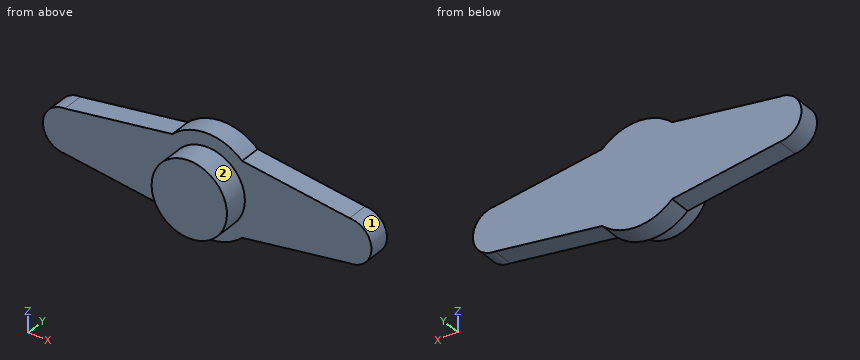
```python
from build123d import *

# Parameters (mm, degrees)
BOSS_EXTRUDE1_DEPTH = 2.54
SKETCH2_R           = 4.3688
BOSS_EXTRUDE2_DEPTH = 2.921


with BuildPart() as part:
    # Sketch1 → Boss-Extrude1 (new body)
    with BuildSketch(Plane(origin=(0, 0, 0), x_dir=(1, 0, 0), z_dir=(0, 1, 0))):
        with BuildLine():
            Line((4.047217222, 4.318), (16.51, 2.54))
            ThreePointArc((16.51, 2.54), (19.05, 0), (16.51, -2.54))
            Line((16.51, -2.54), (4.047217222, -4.318))
            ThreePointArc((4.047217222, -4.318), (0, -5.9182), (-4.047217222, -4.318))
            Line((-4.047217222, -4.318), (-16.51, -2.54))
            ThreePointArc((-16.51, -2.54), (-19.05, 0), (-16.51, 2.54))
            Line((-16.51, 2.54), (-4.047217222, 4.318))
            ThreePointArc((-4.047217222, 4.318), (0, 5.9182), (4.047217222, 4.318))
        make_face()
    extrude(amount=BOSS_EXTRUDE1_DEPTH)

    # Sketch2 → Boss-Extrude2 (add)
    with BuildSketch(Plane.XZ):
        with Locations(Location((0, 0, 0), (0, 0, 270))):
            Circle(SKETCH2_R)
    extrude(amount=BOSS_EXTRUDE2_DEPTH)


solid = part.part
```
For this review, take the finished solid that the model builds, in its own axes (mm). Face numbers are marked on the shaded views. A direction names the side the tool comes from. Round coordinates to 2 decimals unless told otherwise and drop trailing zeros. Write each loop counter-clockwise with the first axis right and the second up, starting at its lowest first coordinate (ties: lowest second). Pieces come first, ordered by that corner, then holes. Notation, with made-up numbers: (37.25, -7.75) - (87.25, -7.75) arc R23 cw to (87.25, 26.25) - close; hole circle Ø2 at (70.5, -27). An arc over 180 degrees is marked (long way). Answer as a JSON object with one key per item and string values.
1. We need section B-B on x = 0. Give the boundary of the cut face in (y, z).
Response values:
{"outline": "(-2.92, -4.37) - (0, -4.37) - (0, -5.92) - (2.54, -5.92) - (2.54, 5.92) - (0, 5.92) - (0, 4.37) - (-2.92, 4.37) - close"}
2. We need section A-A on y = 1.9. Give the boundary of the cut face in (x, z), then the cut area to 3 significant figures.
Response values:
{"outline": "(-16.51, -2.54) - (-4.05, -4.32) arc R5.92 ccw to (4.05, -4.32) - (16.51, -2.54) arc R2.54 ccw to (16.51, 2.54) - (4.05, 4.32) arc R5.92 ccw to (-4.05, 4.32) - (-16.51, 2.54) arc R2.54 ccw to start", "area": "279 mm2"}
3. We need section C-C on z = -4.75. Give the boundary of the cut face in (x, y), then the cut area to 3 significant figures.
Response values:
{"outline": "(-3.53, 0) - (3.53, 0) - (3.53, 2.54) - (-3.53, 2.54) - close", "area": "17.9 mm2"}
4. For pin 1 Ø3.5 at (x, z) = (7, 2) entering from -Y; pin 2 Ø1 at (x, y) = (4, -1) entering from -Z; pin 3 Ø1.5 at (y, z) = (1.5, 2.5) entering from +X, all flat-tipped, find the tip position at first contact; note any pin that passes through.
Response values:
{"pin 1": "stops at y = 0", "pin 2": "stops at z = -2.61", "pin 3": "stops at x = 18.35"}
5. We need section D-D on y = -2.05. Give the boundary of the cut face in (x, z), then the cut area to 3 significant figures.
Response values:
{"outline": "circle Ø8.74 at (0, 0)", "area": "60.0 mm2"}
6. Tool access review of the marked faces 1 and 2: name each direction out of +Z, -Z, +X, -X, +Y, -Y from which nothing blocks a thin tool from reaching the whole face with its end or side.
Response values:
{"face 1": "+X, +Y, -Y", "face 2": "-Y"}
7. To check wall thickness, follow line 1 along X through (y, z) = (-0.15, 0.25); line 2 along Y through (x, z) = (-15, 1.75); line 3 along Z through (x, y) = (3, -2.5). State the ranges of each line that lie inside material, in increasing order.
Response values:
{"line 1": "x = -4.36 to 4.36", "line 2": "y = 0 to 2.54", "line 3": "z = -3.18 to 3.18"}
